from build123d import *

# Parameters (mm, degrees)
SKETCH2_R           = 14
SKETCH2_R_2         = 9
BOSS_EXTRUDE1_DEPTH = 9
FILLET1_R           = 3.875
CUT_EXTRUDE1_START  = -3.875
SKETCH3_R           = 15.875
SKETCH3_R_2         = 11
CUT_EXTRUDE1_DEPTH  = 1.25


with BuildPart() as part:
    # Sketch2 → Boss-Extrude1 (new body)
    with BuildSketch(Plane(origin=(0, 0, 0), x_dir=(1, 0, 0), z_dir=(0, 1, 0))):
        Circle(SKETCH2_R)
        Circle(SKETCH2_R_2, mode=Mode.SUBTRACT)
    extrude(amount=BOSS_EXTRUDE1_DEPTH)

    # Fillet1
    fillet1_edges = [part.edges().sort_by_distance(p)[0] for p in [
        (-14, 0, 0),
        (-14, 9, 0),
    ]]
    fillet(fillet1_edges, radius=FILLET1_R)

    # Sketch3 → Cut-Extrude1 (cut)
    with BuildSketch(Plane(origin=(0, 9, 0), x_dir=(1, 0, 0), z_dir=(0, 1, 0)).offset(CUT_EXTRUDE1_START)):
        Circle(SKETCH3_R)
        Circle(SKETCH3_R_2, mode=Mode.SUBTRACT)
    extrude(amount=-CUT_EXTRUDE1_DEPTH, mode=Mode.SUBTRACT)


solid = part.part
Work out the finished part from the listing and answer in its coordinate system (mm). A direction names the side the tool comes from. Give positions to 0.01 mm unless a question says otherwise; leave off trailing zeros. Order: outer loops, then holes, each group sorted by start corner. A loop starts at its lowest first (then second) coordinate and runs counter-clockwise, first axis right, second up. Notation, with made-up numbers: (-14, 30.5) -> (-4, 30.5) arc R31 ccw to (-4, 61.5) -> close; hole circle Ø5 at (85, 32). An arc over 180 degrees is marked (long way). One line per item, written item: value.
Item 1: Find section A-A, the plane x = 0. Give the vertices of the cut face in (y, z) (3 decimals).
Answer sheet:
outline: (0, -10.125) arc R3.875 ccw to (3.875, -14) -> (3.875, -11) -> (5.125, -11) -> (5.125, -14) arc R3.875 ccw to (9, -10.125) -> (9, -9) -> (0, -9) -> close; (0, 9) -> (9, 9) -> (9, 10.125) arc R3.875 ccw to (5.125, 14) -> (5.125, 11) -> (3.875, 11) -> (3.875, 14) arc R3.875 ccw to (0, 10.125) -> close
Item 2: A tool of negligible diameter and unlimited length cuts with its end or side. For faces 1 (the flat face through (6.2, 3.875, 9.3)), 2 (the flat face through (-7, 0, 6)), from which of +Z, -Z, +X, -X, +Y, -Y can it reach the whole face along a straight path? Write none if from no direction.
Answer sheet:
face 1: none
face 2: +Z, -Z, +X, -X, -Y
Item 3: Straight lines are drawn through the part: probe 1 along X at (y, z) = (5.25, 0); probe 2 along Y at (x, z) = (-11.25, 4.75) (3 decimals); probe 3 along Z at (x, y) = (5.5, 2). For each, find the intervals that lie inside material, in ascending order.
Answer sheet:
probe 1: -14 to -9, 9 to 14
probe 2: 0.61 to 3.875, 5.125 to 8.39
probe 3: -12.35 to -7.12, 7.12 to 12.35
Item 4: Flat-ended cylindrical pins translate along their axes: P1, Ø2, axis at x = 6.5, y = 5.5, coming from the +Z side; P2, Ø5, axis at y = 8, z = 0, coming from the -X side; P3, Ø1, axis at x = -5, y = 2, coming from the -Z side; P4, Ø8.5, axis at x = 3.5, z = -6, coming from the +Y side. Find the tip coordinate at first contact, or state that the pin passes through.
Answer sheet:
P1: z = 12.86
P2: x = -13.98
P3: z = -12.88
P4: y = 9
Item 5: Find section C-C, the plane y = 2.5. Give the vertices of the cut face in (x, z).
Answer sheet:
outline: circle Ø27.5 at (0, 0); hole circle Ø18 at (0, 0)
Item 6: Find section B-B, the plane z = 0. Give the vertices of the cut face in (x, y) (3 decimals), plus the area to 3 significant figures.
Answer sheet:
outline: (-14, 3.875) arc R3.875 ccw to (-10.125, 0) -> (-9, 0) -> (-9, 9) -> (-10.125, 9) arc R3.875 ccw to (-14, 5.125) -> (-11, 5.125) -> (-11, 3.875) -> close; (9, 0) -> (10.125, 0) arc R3.875 ccw to (14, 3.875) -> (11, 3.875) -> (11, 5.125) -> (14, 5.125) arc R3.875 ccw to (10.125, 9) -> (9, 9) -> close
area: 69.6 mm²
Item 7: Determine the mould class of faces 3 (the cylindrical face through (-1.172, 4.437, -8.923)), 4 (the flat face through (-7, 9, 6)), 5 (the cylindrical face through (-2.38, 4.51, 10.74)) for opening direction Z: released by +Z, released by -Z, zero draft, split by the parting line, or undercut.
Answer sheet:
face 3: undercut
face 4: zero draft
face 5: split by the parting line
